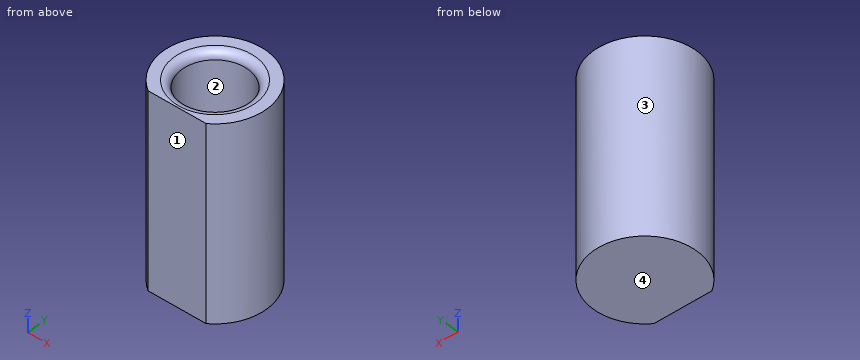
from build123d import *

# Parameters (mm, degrees)
F0_R     = 4.25
F1_DEPTH = 14
F2_DEPTH = 25
F3_R     = 1


with BuildPart() as f1:
    # F0 (on Top) → F1 (new body)
    with BuildSketch(Plane.XY):
        Circle(F0_R)
    extrude(amount=F1_DEPTH)

    # F0 (on Top) → F2 (join)
    with BuildSketch(Plane.XY):
        with BuildLine():
            Line((-3.737981, -5.5), (3.737981, -5.5))
            ThreePointArc((3.737981, -5.5), (0, 6.65), (-3.737981, -5.5))
        make_face()
        Circle(F0_R, mode=Mode.SUBTRACT)
    extrude(amount=F2_DEPTH)

    # F3
    f3_edges = [f1.edges().sort_by_distance(p)[0] for p in [
        (-4.25, 0, 14),
        (-4.25, 0, 25),
    ]]
    fillet(f3_edges, radius=F3_R)


solid = f1.part
Input: part model. Units: mm. Frame: model coordinates. Face numbers are marked on the shaded views. Give positions to 0.01 mm unless a question says otherwise; leave off trailing zeros. Write each loop counter-clockwise with the first axis right and the second up, starting at its lowest first coordinate (ties: lowest second). Pieces come first, ordered by that corner, then holes. Notation, with made-up numbers: M 44,73 L 57,73 A16 cw 57,88 Z; hole C -9,-26.75 d10. An arc over 180 degrees is marked long. Write item = value, one per line. Start each with the question number.
1) Cut plane D-D on z = 4.5. Return the cut outline in (x, y), then the cut area to 3 significant figures.
2) Material intervals for line 1 along X through (y, z) = (0.5, 21); line 2 along Y through (x, z) = (-0.25, 22.5); line 3 along Z through (x, y) = (-2, -2), sorted ascending. Write a range as [from, to].
3) Cut plane A-A on x = 0. Return the cut outline in (y, z), then the cut area to 3 significant figures.
4) First-contact query: pin 1 Ø1.5 at (x, y) = (-1.5, -1) entering from +Z; pin 2 Ø1 at (y, z) = (-3, 21.5) entering from +X. Flat tips, straight axial feed; report the tip coordinate or a pass-through.
5) Draft query along Y for the marked faces 1, 2, 3 and 4. Return one class per face: +Y half, -Y half, draft (parallel to the pull), parting line (faces both ways), or undercut.
6) Cut plane B-B on y = 0. Return the cut outline in (x, z).
7) Cut plane C-C on z = 18.25. Return the cut outline in (x, y).
Solved:
q1.outline = M -3.74,-5.5 L 3.74,-5.5 A6.65 ccw long Z
q1.area = 133 mm2
q2.line_1 = [-6.63, -4.22], [4.22, 6.63]
q2.line_2 = [-5.5, -4.24], [4.24, 6.65]
q2.line_3 = [0, 14]
q3.outline = M -5.5,0 L 6.65,0 L 6.65,25 L 5.25,25 A1 ccw 4.25,24 L 4.25,15 A1 cw 3.25,14 L -3.25,14 A1 cw -4.25,15 L -4.25,24 A1 ccw -5.25,25 L -5.5,25 Z
q3.area = 210 mm2
q4.pin_1 = 14
q4.pin_2 = 6.16
q5.face_1 = -Y half
q5.face_2 = undercut
q5.face_3 = parting line
q5.face_4 = draft
q6.outline = M -6.65,0 L 6.65,0 L 6.65,25 L 5.25,25 A1 ccw 4.25,24 L 4.25,15 A1 cw 3.25,14 L -3.25,14 A1 cw -4.25,15 L -4.25,24 A1 ccw -5.25,25 L -6.65,25 Z
q7.outline = M -3.74,-5.5 L 3.74,-5.5 A6.65 ccw long Z; hole C 0,0 d8.5
